Input: dimensioned drawing with shaded views. Units: mm. Origin: part minimum x, y, z. A direction names the side the tool comes from. Round coordinates to 2 decimals unless told otherwise and drop trailing zeros. Loops run counter-clockwise (first coordinate to the right, second up) from the corner with the lowest first, then second, coordinate; pieces in that order, holes last.
1) Draft query along Y for the marked faces 6, 7 and 8. Return one class per face: pulls with the +Y half, pulls with the -Y half, needs draft (parallel to the pull), parting line crosses it, or undercut.
2) Ray query, line 1 along X through (y, z) = (22, 16.5); line 2 along X through (y, z) = (28.5, 28.5); line 3 along Z through (x, y) = (27.5, 35). Return the intervals inside material, ascending.
3) Section B-B, the plane z = 11. Return loops of the section in (x, y).
4) First-contact query: pin 1 (18 mm diameter, centred on x = 29.5, y = 12.5, fed in from +Z); pin 2 (12 mm diameter, centred on x = 49.5, z = 19, fed in from -Y); pin 3 (18.5 mm diameter, centred on y = 11, z = 28, fed in from +X). Flat tips, straight axial feed; report the tip coordinate or a pass-through.
5) Section C-C, the plane y = 47. Return loops of the section in (x, z).
6) Section A-A, the plane x = 7.5. Return loops of the section in (y, z), and give its area (3 significant figures).
7) Section D-D, the plane x = 15.5. Return loops of the section in (y, z).
8) Access query for the marked faces 1, 2, 3, 4 and 5. Directions: +Z, -Z, +X, -X, +Y, -Y. A direction counts if a zero-diameter tool reaches every point of the face in a straight line with its end or side. Return the directions, or none.
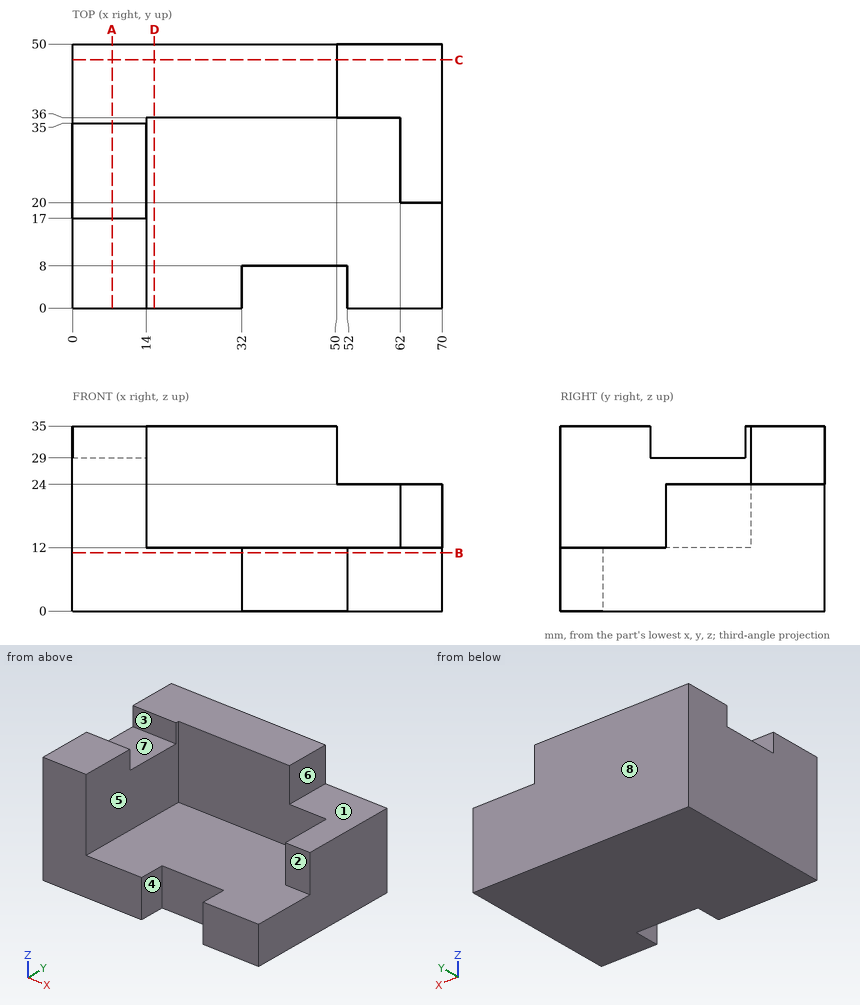
Final values:
1. face 6: needs draft
1. face 7: undercut
1. face 8: pulls with the +Y half
2. line 1: x = 0 to 14, 62 to 70
2. line 2: x = 0 to 14
2. line 3: z = 0 to 12
3. outline: (0, 0) - (32, 0) - (32, 8) - (52, 8) - (52, 0) - (70, 0) - (70, 50) - (0, 50) - close
4. pin 1: stops at z = 12
4. pin 2: stops at y = 36
4. pin 3: stops at x = 14
5. outline: (0, 0) - (70, 0) - (70, 24) - (50, 24) - (50, 35) - (0, 35) - close
6. outline: (0, 0) - (50, 0) - (50, 35) - (35, 35) - (35, 29) - (17, 29) - (17, 35) - (0, 35) - close
6. area: 1,640 mm2
7. outline: (0, 0) - (50, 0) - (50, 35) - (36, 35) - (36, 12) - (0, 12) - close
8. face 1: +Z, +X, +Y, -Y
8. face 2: +Z, +X, -Y
8. face 3: +Z, +X, -X
8. face 4: +Z, -Z, -Y
8. face 5: +Z, -Y
